For this review, take the finished solid that the model builds, in its own axes (mm). A direction names the side the tool comes from. Round coordinates to 2 decimals unless told otherwise and drop trailing zeros. Loops run counter-clockwise (first coordinate to the right, second up) from the corner with the lowest first, then second, coordinate; pieces in that order, holes last.
1. Clearance check with flat-ended pins moving along their axes: pin 1 Ø2 at (x, y) = (2, 2) entering from -Z; pin 2 Ø5 at (x, y) = (-4, 10) entering from +Z. State where each tip first meets the part, or that it passes through.
2. Consider section B-B on y = 14. State the section outline as (x, z) points.
3. Draft analysis for pull direction X (two halves, no side actions). For faces 3 (the cylindrical face through (0.077, -17.034, -2.117)), 4 (the flat face through (-6.5, 5, 0)), 5 (the cylindrical face through (-5.99, -8.04, 19.4)), state which applies: released by +X, released by -X, zero draft, split by the parting line, or undercut.
4. Consider section A-A on y = 1. State the section outline as (x, z) points, then the cut area to 3 significant figures.
5. To check wall thickness, follow line 1 along Z through (x, y) = (1.25, -16); line 2 along Y through (x, z) = (3.25, 0) (3 decimals); line 3 along Z through (x, y) = (-2.5, 17). State the ranges of each line that lie inside material, in increasing order.
6. Tool access review of faces 1 (the cylindrical face through (0.08, 9.17, -14.51)), 2 (the cylindrical face through (6.01, -8.04, 19.4)): name each direction out of +Z, -Z, +X, -X, +Y, -Y from which nothing blocks a thin tool from reaching the whole face with its end or side.
from build123d import *

# Parameters (mm, degrees)
SKETCH_3_OUTSIDE_W        = 52.04
SKETCH_3_OUTSIDE_H        = 52.04
CUT_EXTRUDE_3_DEPTH       = 5.5
PATTERN_CIRCULAR_2_COUNT  = 25
SKETCH_7_R                = 5
CUT_EXTRUDE_4_DEPTH       = 36.616007637
CUT_EXTRUDE_25_DEPTH      = 33.810059433
CUT_EXTRUDE_25_DEPTH_BACK = 33.810059433
SKETCH_42_W               = 11.690908627
SKETCH_42_H               = 55.464155105
SKETCH_42_W_2             = 17.903263655
SKETCH_42_H_2             = 55.986187397
CUT_EXTRUDE_27_DEPTH      = 35.372954485
CUT_EXTRUDE_27_DEPTH_BACK = 35.372954485
SKETCH_43_R               = 22.5
SKETCH_43_R_2             = 21
SKETCH_44_R               = 5
SKETCH_44_R_2             = 4.7
EXTRUDE_1_DEPTH           = 13


with BuildPart() as part:
    # 草图1 → 旋转1 (revolve)
    with BuildSketch(Plane.XY, mode=Mode.PRIVATE) as revolve_1_sk:
        Polygon((-8, 15), (-5.5, 15), (-5.5, 19.325), (5.5, 19.325), (5.5, 15), (8, 15), (8, 0), (-8, 0), align=None)
    revolve(revolve_1_sk.sketch.rotate(Axis((-8, 0, 0), (1, 0, 0)), 90), axis=Axis((-8, 0, 0), (1, 0, 0)))

    # 草图3 outside → 切除-拉伸3 (cut, symmetric)
    with BuildSketch(Plane(origin=(0, 0, 0), x_dir=(0, 0, -1), z_dir=(1, 0, 0))):
        Rectangle(SKETCH_3_OUTSIDE_W, SKETCH_3_OUTSIDE_H)
        with BuildLine():
            ThreePointArc((-2.114672063, 19.208950702), (0, -19.325), (2.114672063, 19.208950702))
            ThreePointArc((2.114672063, 19.208950702), (1.727490621, 19.085403384), (1.559968713, 18.715119953))
            ThreePointArc((1.559968713, 18.715119953), (0, 17.165), (-1.559968713, 18.715119953))
            ThreePointArc((-1.559968713, 18.715119953), (-1.727490621, 19.085403384), (-2.114672063, 19.208950702))
        make_face(mode=Mode.SUBTRACT)
    cut_extrude_3 = extrude(amount=CUT_EXTRUDE_3_DEPTH, both=True, mode=Mode.SUBTRACT)

    # 阵列(圆周)2: 切除-拉伸3 ×25 about axis
    pattern_circular_2_axis = Axis((0, 0, 0), (1, 0, 0))
    for i in range(1, PATTERN_CIRCULAR_2_COUNT):
        add(cut_extrude_3.rotate(pattern_circular_2_axis, i * 360 / PATTERN_CIRCULAR_2_COUNT), mode=Mode.SUBTRACT)

    # 草图4 → 旋转2 (revolve)
    with BuildSketch(Plane.XY, mode=Mode.PRIVATE) as revolve_2_sk:
        Polygon((-7, 22.5), (-7, 15), (-5.5, 15), (-5.5, 21), (-5.901923789, 22.5), align=None)
        Polygon((7, 22.5), (7, 15), (5.5, 15), (5.5, 21), (5.901923789, 22.5), align=None)
    revolve(revolve_2_sk.sketch.rotate(Axis((-8, 0, 0), (1, 0, 0)), 180), axis=Axis((-8, 0, 0), (1, 0, 0)))

    # 草图7 → 切除-拉伸4 (cut, through all)
    with BuildSketch(Plane.ZY.offset(8)):
        Circle(SKETCH_7_R)
    extrude(amount=-CUT_EXTRUDE_4_DEPTH, mode=Mode.SUBTRACT)

    # 草图42 → 切除-拉伸25 (cut, two sides: drawn at the far end of the back side and taken through both)
    with BuildSketch(Plane(origin=(0, 0, 0), x_dir=(1, 0, 0), z_dir=(0, 1, 0)).offset(-CUT_EXTRUDE_25_DEPTH_BACK)):
        with Locations((-12.345454314, 2.796156441)):
            Rectangle(SKETCH_42_W, SKETCH_42_H)
        with Locations((15.451631827, 4.731003793)):
            Rectangle(SKETCH_42_W_2, SKETCH_42_H_2)
    extrude(amount=CUT_EXTRUDE_25_DEPTH + CUT_EXTRUDE_25_DEPTH_BACK, mode=Mode.SUBTRACT)

    # 草图43 → 切除-拉伸27 (cut, two sides: drawn at the far end of the back side and taken through both)
    with BuildSketch(Plane.ZY.offset(6.5).offset(-CUT_EXTRUDE_27_DEPTH_BACK)):
        Circle(SKETCH_43_R)
        Circle(SKETCH_43_R_2, mode=Mode.SUBTRACT)
    extrude(amount=CUT_EXTRUDE_27_DEPTH + CUT_EXTRUDE_27_DEPTH_BACK, mode=Mode.SUBTRACT)

    # 草图44 → 凸台-拉伸1 (add)
    with BuildSketch(Plane.ZY.offset(6.5)):
        Circle(SKETCH_44_R)
        Circle(SKETCH_44_R_2, mode=Mode.SUBTRACT)
    extrude(amount=-EXTRUDE_1_DEPTH)


solid = part.part
Resolved:
1. pin 1: stops at z = -18.99
1. pin 2: stops at z = 19.42
2. outline: (-6.5, -15.65) - (-5.5, -15.65) - (-5.5, -11.3) - (5.5, -11.3) - (5.5, -15.65) - (6.5, -15.65) - (6.5, 15.65) - (5.5, 15.65) - (5.5, 11.3) - (-5.5, 11.3) - (-5.5, 15.65) - (-6.5, 15.65) - close
3. face 3: undercut
3. face 4: released by -X
3. face 5: zero draft
4. outline: (-6.5, -20.98) - (-5.5, -20.98) - (-5.5, -17.14) - (5.5, -17.14) - (5.5, -20.98) - (6.5, -20.98) - (6.5, -4.59) - (-6.5, -4.59) - close; (-6.5, 4.59) - (6.5, 4.59) - (6.5, 20.98) - (5.5, 20.98) - (5.5, 17.14) - (-5.5, 17.14) - (-5.5, 20.98) - (-6.5, 20.98) - close
4. area: 342 mm2
5. line 1: z = -9.7 to -7.56, -6.23 to 6.23, 7.56 to 9.7
5. line 2: y = -19.325 to -4.7, 4.7 to 17.165
5. line 3: z = -7.58 to -5.73, -3.59 to 3.59, 5.73 to 7.58
6. face 1: none
6. face 2: +X, -X
